from build123d import *

# Parameters (mm, degrees)
BOSS_EXTRUDE1_DEPTH = 10
CUT_EXTRUDE38_DEPTH = 10


with BuildPart() as part:
    # Sketch1 → Boss-Extrude1 (new body)
    with BuildSketch(Plane.XY):
        with BuildLine():
            Line((-50, 60), (50, 60))
            ThreePointArc((50, 60), (57.071067812, 57.071067812), (60, 50))
            Line((60, 50), (60, -50))
            ThreePointArc((60, -50), (57.071067812, -57.071067812), (50, -60))
            Line((50, -60), (-50, -60))
            ThreePointArc((-50, -60), (-57.071067812, -57.071067812), (-60, -50))
            Line((-60, -50), (-60, 50))
            ThreePointArc((-60, 50), (-57.071067812, 57.071067812), (-50, 60))
        make_face()
    extrude(amount=BOSS_EXTRUDE1_DEPTH)

    # Sketch2 → Cut-Extrude38 (cut)
    with BuildSketch(Plane.XY.offset(10)):
        Polygon((-37.794871795, 50), (-17.822916667, 50), (0.025641026, 14.923878205), (17.874198718, 50), (37.846153846, 50), (9, -6.690705128), (9, -50), (-8.948717949, -50), (-8.948717949, -6.690705128), align=None)
    extrude(amount=-CUT_EXTRUDE38_DEPTH, mode=Mode.SUBTRACT)


solid = part.part
Verification items for the finished model (mm, model axes). A direction names the side the tool comes from. Coordinates: 2 decimals unless noted, no trailing zeros. Write each loop counter-clockwise with the first axis right and the second up, starting at its lowest first coordinate (ties: lowest second). Pieces come first, ordered by that corner, then holes. Notation, with made-up numbers: M -34,88 L -23,88 A30 cw -23,112 Z; hole C 53.5,80 d9. An arc over 180 degrees is marked long. Use CSV: the item, a comma, the result in double quotes.
Q1. Set-up check for faces 4 (the flat face through (14, 1, 10)), 5 (the flat face through (-8.949, -29, 5)): record each of +Z, -Z, +X, -X, +Y, -Y from which the full face is reachable in a straight line by a thin tool's end or side.
Computed values:
face 4,"+Z, +X, -X, +Y, -Y"
face 5,"+Z, -Z"
Q2. Mould release check, pull along Y, two halves, no side actions. Record for faces 1 (the flat face through (9, -28, 5)), 2 (the cylindrical face through (-57.15, 56.99, 4.93)), 3 (the flat face through (-60, -1, 5)): pulls with the +Y half, pulls with the -Y half, needs draft (parallel to the pull), parting line crosses it, or undercut.
Computed values:
face 1,"undercut"
face 2,"pulls with the +Y half"
face 3,"needs draft"
Q3. Thickness scan on line 1 along X through (y, z) = (32.5, 7.5); line 2 along X through (y, z) = (47.5, 6.25); line 3 along X through (y, z) = (-37, 7.75). Record the ranges inside material, lowest first. Write a range as [from, to].
Computed values:
line 1,"[-60, -28.89], [-8.92, 8.97], [28.94, 60]"
line 2,"[-60, -36.52], [-16.55, 16.6], [36.57, 60]"
line 3,"[-60, -8.95], [9, 60]"
Q4. Section check C-C, the plane y = 27. Enter the section's corners in (x, z), and give its area (3 significant figures).
Computed values:
outline,"M -60,0 L -26.09,0 L -26.09,10 L -60,10 Z; M -6.12,0 L 6.17,0 L 6.17,10 L -6.12,10 Z; M 26.14,0 L 60,0 L 60,10 L 26.14,10 Z"
area,"801 mm²"
Q5. Section check D-D, the plane x = 5.5. Enter the section's corners in (y, z), and give its area (3 significant figures).
Computed values:
outline,"M -60,0 L -50,0 L -50,10 L -60,10 Z; M 25.68,0 L 60,0 L 60,10 L 25.68,10 Z"
area,"443 mm²"
Q6. Section check B-B, the plane x = -12. Enter the section's corners in (y, z).
Computed values:
outline,"M -60,0 L -0.69,0 L -0.69,10 L -60,10 Z; M 38.56,0 L 60,0 L 60,10 L 38.56,10 Z"
Q7. Section check A-A, the plane z = 8. Enter the section's corners in (x, y), and give its area (3 significant figures).
Computed values:
outline,"M -60,-50 A10 ccw -50,-60 L 50,-60 A10 ccw 60,-50 L 60,50 A10 ccw 50,60 L -50,60 A10 ccw -60,50 Z; hole M -37.79,50 L -8.95,-6.69 L -8.95,-50 L 9,-50 L 9,-6.69 L 37.85,50 L 17.87,50 L 0.03,14.92 L -17.82,50 Z"
area,"11,500 mm²"
